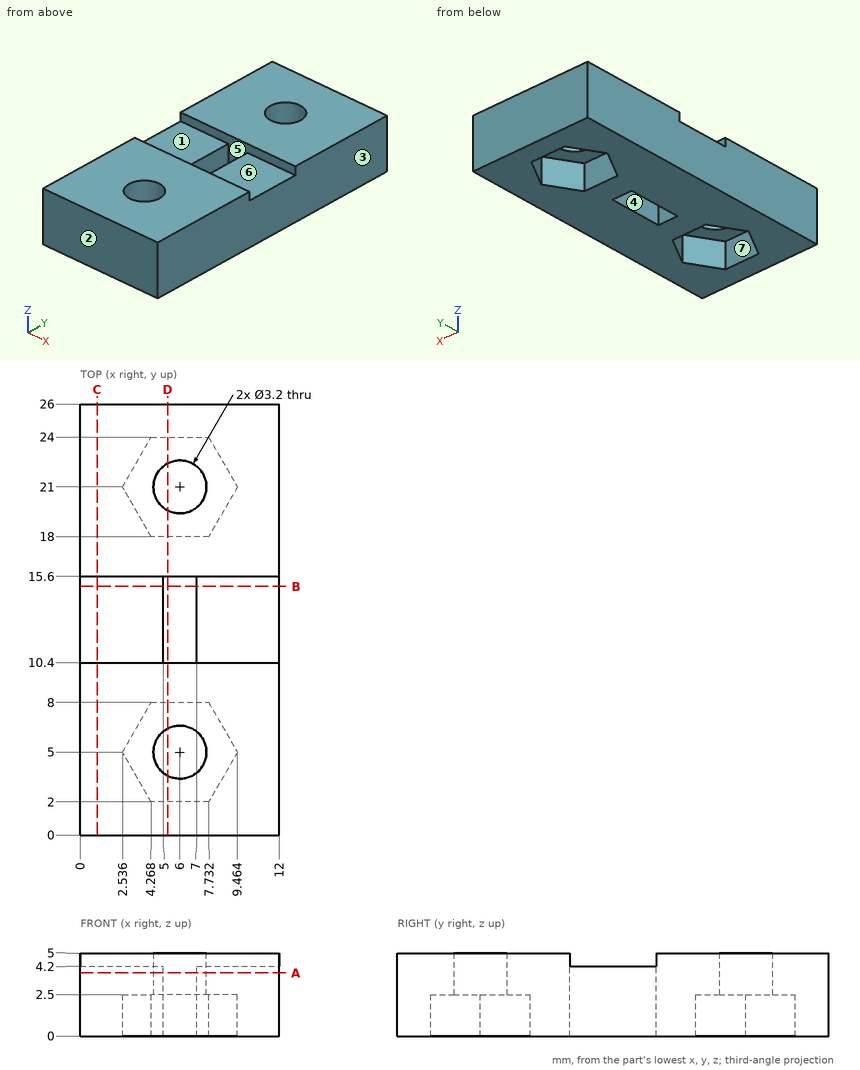
Geometry: see drawing. Coordinates: mm, zero at the bounding-box minimum. A direction names the side the tool comes from. Round coordinates to 2 decimals unless told otherwise and drop trailing zeros. Order: outer loops, then holes, each group sorted by start corner. A loop starts at its lowest first (then second) coordinate and runs counter-clockwise, first axis right, second up. Notation, with made-up numbers: (86, 87) -> (136, 87) arc R13 cw to (136, 93) -> close; hole circle Ø2 at (-16.5, -20.5). An arc over 180 degrees is marked (long way). Answer as CSV lines item,"result".
Item 1: Pull-direction query (Y, two-part tool) for the marked faces 1, 2 and 3; classes: pulls with the +Y half, pulls with the -Y half, needs draft (parallel to the pull), parting line crosses it, or undercut.
A:
face 1,"undercut"
face 2,"pulls with the -Y half"
face 3,"needs draft"
Item 2: Section C-C, the plane x = 1. Return loops of the section in (y, z).
A:
outline,"(0, 0) -> (26, 0) -> (26, 5) -> (15.6, 5) -> (15.6, 4.2) -> (10.4, 4.2) -> (10.4, 5) -> (0, 5) -> close"
Item 3: Section A-A, the plane z = 3.8. Return loops of the section in (x, y).
A:
outline,"(0, 0) -> (12, 0) -> (12, 26) -> (0, 26) -> close; hole circle Ø3.2 at (6, 5); hole circle Ø3.2 at (6, 21); hole (5, 10.4) -> (7, 10.4) -> (7, 15.6) -> (5, 15.6) -> close"
Item 4: Pin query (flat end, axial travel): pin 1 Ø3.5 at (x, y) = (6, 21) entering from -Z. Return the tip coordinate at first contact, or that it passes through.
A:
pin 1,"z = 2.5"
Item 5: Reachability of the marked faces 4, 5, 6 and 7 from +Z, -Z, +X, -X, +Y, -Y: full face, straight path, thin tool, end or side. Return the list, or none.
A:
face 4,"+Z, -Z"
face 5,"+Z"
face 6,"+Z, +X, -X"
face 7,"-Z"
Item 6: Section D-D, the plane x = 5.25. Return loops of the section in (y, z).
A:
outline,"(0, 0) -> (2, 0) -> (2, 2.5) -> (3.59, 2.5) -> (3.59, 5) -> (0, 5) -> close; (6.41, 2.5) -> (8, 2.5) -> (8, 0) -> (10.4, 0) -> (10.4, 5) -> (6.41, 5) -> close; (15.6, 0) -> (18, 0) -> (18, 2.5) -> (19.59, 2.5) -> (19.59, 5) -> (15.6, 5) -> close; (22.41, 2.5) -> (24, 2.5) -> (24, 0) -> (26, 0) -> (26, 5) -> (22.41, 5) -> close"
Item 7: Line query: L1, parallel to Y at x = 6, z = 4.1; L2, parallel to Y at x = 6.75, z = 1.15; L3, parallel to X at y = 5, z = 3.6. Output: solid intervals per line, ascending.
A:
L1,"0 to 3.4, 6.6 to 10.4, 15.6 to 19.4, 22.6 to 26"
L2,"0 to 2, 8 to 10.4, 15.6 to 18, 24 to 26"
L3,"0 to 4.4, 7.6 to 12"
Item 8: Section B-B, the plane y = 15. Return loops of the section in (x, z).
A:
outline,"(0, 0) -> (5, 0) -> (5, 4.2) -> (0, 4.2) -> close; (7, 0) -> (12, 0) -> (12, 4.2) -> (7, 4.2) -> close"
